For this review, take the finished solid that the model builds, in its own axes (mm). A direction names the side the tool comes from. Coordinates: 2 decimals unless noted, no trailing zeros. Loops run counter-clockwise (first coordinate to the right, second up) from the corner with the lowest first, then second, coordinate; pieces in that order, holes last. Notation, with made-up numbers: M 28.25,6 L 76.25,6 A20 cw 76.25,23 Z; hole C 18,28 d11. An arc over 180 degrees is marked long. Answer as a JSON object with one key per item and string values. Group by question number.
Item 1: Add section B-B (x = 0). State the section outline as (y, z) points, then the cut area to 3 significant figures.
Item 2: Add section A-A (z = -27). State the section outline as (x, y) points, then the cut area to 3 significant figures.
Item 3: Mouldability with a two-part tool opening along Y and no side actions: class faces 3 (the face through (15, -5, 14)), 4 (the face through (0, -10, 0)), 5 (the face through (-19.524, 2.605, -4.336)), 6 (the face through (9.76, 12.46, 31)) as +Y half, -Y half, draft (parallel to the pull), parting line (faces both ways), or undercut.
Item 4: Insertion check: pin 1 (5 mm diameter, centred on x = 22, y = -3, fed in from -Z); pin 2 (6 mm diameter, centred on y = 12, z = 20.5, fed in from +X); pin 3 (2 mm diameter, centred on x = -5, y = -3, fed in from -Z). Each pin has a flat end and moves straight along its axis. Give the tip position at first contact, or say it passes through.
Item 5: Wall thickness on L1, parallel to Y at x = -6, z = -26; L2, parallel to Z at x = 14, y = 8; L3, parallel to X at y = 3.5, z = -17: over which ranges is each line inside the solid? List them lowest first. Write a range as from..to.
Item 6: Add section D-D (y = 11.75). State the section outline as (x, z) points.
Item 7: Add section C-C (z = 0). State the section outline as (x, y) points.
Item 8: Tool access review of faces 1 (the face through (9.76, -7.54, 31)), 2 (the face through (15, 10, 14)): name each direction out of +Z, -Z, +X, -X, +Y, -Y from which nothing blocks a thin tool from reaching the whole face with its end or side.
from build123d import *

# Parameters (mm, degrees)
SKETCH1_R           = 20
BOSS_EXTRUDE1_DEPTH = 10
SKETCH2_R           = 32.5
BOSS_EXTRUDE2_DEPTH = 5
BOSS_EXTRUDE3_START = -20
SKETCH2_2_R         = 32.5
BOSS_EXTRUDE3_DEPTH = 5


with BuildPart() as part:
    # Sketch1 → Boss-Extrude1 (new, symmetric)
    with BuildSketch(Plane(origin=(0, 0, 0), x_dir=(1, 0, 0), z_dir=(0, 1, 0))):
        with Locations(Location((0, 0, 0), (0, 0, 270))):
            Circle(SKETCH1_R)
    extrude(amount=BOSS_EXTRUDE1_DEPTH, both=True)

    # Sketch2 → Boss-Extrude2 (add)
    with BuildSketch(Plane(origin=(0, 10, 0), x_dir=(1, 0, 0), z_dir=(0, 1, 0))):
        with Locations(Location((0, 0, 0), (0, 0, 270))):
            Circle(SKETCH2_R)
    extrude(amount=BOSS_EXTRUDE2_DEPTH)

    # Sketch2<2> → Boss-Extrude3 (add)
    with BuildSketch(Plane(origin=(0, 10, 0), x_dir=(1, 0, 0), z_dir=(0, 1, 0)).offset(BOSS_EXTRUDE3_START)):
        with Locations(Location((0, 0, 0), (0, 0, 270))):
            Circle(SKETCH2_2_R)
    extrude(amount=BOSS_EXTRUDE3_DEPTH)


solid = part.part
From the geometry:
{
 "1": {"outline": "M -10,-32.5 L -5,-32.5 L -5,-20 L 10,-20 L 10,-32.5 L 15,-32.5 L 15,32.5 L 10,32.5 L 10,20 L -5,20 L -5,32.5 L -10,32.5 Z", "area": "1,250 mm²"},
 "2": {"outline": "M -18.09,-10 L 18.09,-10 L 18.09,-5 L -18.09,-5 Z; M -18.09,10 L 18.09,10 L 18.09,15 L -18.09,15 Z", "area": "362 mm²"},
 "3": {"face 3": "undercut", "face 4": "-Y half", "face 5": "undercut", "face 6": "draft"},
 "4": {"pin 1": "stops at z = -25.22", "pin 2": "stops at x = 27.39", "pin 3": "stops at z = -19.6"},
 "5": {"L1": "y = -10..-5, 10..15", "L2": "z = -14.28..14.28", "L3": "x = -10.54..10.54"},
 "6": {"outline": "C 0,0 d65"},
 "7": {"outline": "M -32.5,-10 L 32.5,-10 L 32.5,-5 L 20,-5 L 20,10 L 32.5,10 L 32.5,15 L -32.5,15 L -32.5,10 L -20,10 L -20,-5 L -32.5,-5 Z"},
 "8": {"face 1": "+Y, -Y", "face 2": "none"}
}
